```python
from build123d import *

# Parameters (mm, degrees)
F0_W     = 276
F0_H     = 25
F1_DEPTH = 25
F3_D     = 20
F3_DEPTH = 10
F3_TIP   = 6.0086061903
F4_R     = 5


with BuildPart() as f1:
    # F0 (on Front) → F1 (new body)
    with BuildSketch(Plane.XZ):
        with Locations((71.2675039768, 12.5)):
            Rectangle(F0_W, F0_H)
    extrude(amount=F1_DEPTH)

    # F3
    with Locations(Plane(origin=(0, 0, 0), x_dir=(1, 0, 0), z_dir=(0, 0, -1))):
        with Locations((140.2675039768, 12.5), (71.2675039768, 12.5), (2.2675039768, 12.5)):
            Hole(F3_D / 2, depth=F3_DEPTH)
            with Locations((0, 0, -(F3_DEPTH + F3_TIP / 2))):  # 118° drill point
                Cone(0, F3_D / 2, F3_TIP, mode=Mode.SUBTRACT)

    # F4
    f4_edges = [f1.edges().sort_by_distance(p)[0] for p in [
        (209.267504, -12.5, 25),
        (-66.732496, -12.5, 25),
        (71.267504, 0, 25),
        (71.267504, -25, 25),
        (209.267504, -12.5, 0),
        (209.267504, 0, 12.5),
        (209.267504, -25, 12.5),
        (-66.732496, -12.5, 0),
        (-66.732496, 0, 12.5),
        (-66.732496, -25, 12.5),
    ]]
    fillet(f4_edges, radius=F4_R)


solid = f1.part
```
Input: part model. Units: mm. Frame: model coordinates. A direction names the side the tool comes from. Coordinates: 2 decimals unless noted, no trailing zeros. Write each loop counter-clockwise with the first axis right and the second up, starting at its lowest first coordinate (ties: lowest second). Pieces come first, ordered by that corner, then holes. Notation, with made-up numbers: M -2.75,22.25 L 40.25,22.25 A11 cw 40.25,42.25 Z; hole C -5.5,62 d1. An arc over 180 degrees is marked long. Use one line per item in the form item = value.
Q1. Draft query along X for faces 3 (the face through (-65.307, -23.496, 10.14)), 4 (the face through (62.03, -8.67, 5.07)), 5 (the face through (207.764, -12.605, 23.574)). Return one class per face: released by +X, released by -X, zero draft, split by the parting line, or undercut.
Answer below:
face_3 = released by -X
face_4 = undercut
face_5 = released by +X
Q2. Set-up query: faces 1 (the face through (207.764, -1.426, 10.14)), 2 (the face through (4.44, -2.74, 5.07)). Return all of +Z, -Z, +X, -X, +Y, -Y with unobstructed straight access to the full face (end or side cutting, diameter ignored); none if empty.
Answer below:
face_1 = +Z, -Z, +X, +Y
face_2 = -Z
Q3. Section A-A (x = 154.5). Return loops of the section in (y, z), plus the area to 3 significant figures.
Answer below:
outline = M -25,0 L 0,0 L 0,20 A5 ccw -5,25 L -20,25 A5 ccw -25,20 Z
area = 614 mm²
Q4. First-contact query: pin 1 (1 mm diameter, centred on y = -19, z = 21.5, fed in from +X); pin 2 (1.5 mm diameter, centred on x = 154, y = -21.5, fed in from +Z). Flat tips, straight axial feed; report the tip coordinate or a pass-through.
Answer below:
pin_1 = 209.17
pin_2 = 24.94
Q5. Material intervals for probe 1 along X at (y, z) = (-15.75, 8); probe 2 along X at (y, z) = (-4.75, 7.5); probe 3 along X at (y, z) = (-14.5, 20.5), sorted ascending. Write a range as from..to.
Answer below:
probe_1 = -66.73..-7.19, 11.72..61.81, 80.72..130.81, 149.72..209.27
probe_2 = -66.73..-4.05, 8.59..64.95, 77.59..133.95, 146.59..209.26
probe_3 = -66.71..209.24
